from build123d import *

# Parameters (mm, degrees)
SKETCH_1_W          = 10
SKETCH_1_H          = 10
SKETCH_1_W_2        = 8
SKETCH_1_H_2        = 8
EXTRUDE_1_DEPTH     = 191.5
SKETCH_2_R          = 1.5
CUT_EXTRUDE_1_DEPTH = 11
SKETCH_3_R          = 1.5
CUT_EXTRUDE_2_DEPTH = 11


with BuildPart() as part:
    # 草图1 → 拉伸-薄壁1 (new body)
    with BuildSketch(Plane.XY):
        Rectangle(SKETCH_1_W, SKETCH_1_H)
        Rectangle(SKETCH_1_W_2, SKETCH_1_H_2, mode=Mode.SUBTRACT)
    extrude(amount=EXTRUDE_1_DEPTH)

    # 草图2 → 切除-拉伸1 (cut, through all)
    with BuildSketch(Plane.XZ.offset(5)):
        with Locations((0, 183.994446501)):
            Circle(SKETCH_2_R)
        with Locations((0, 29)):
            Circle(SKETCH_2_R)
        with Locations((0, 173.994446501)):
            Circle(SKETCH_2_R)
        with Locations((0, 100)):
            Circle(SKETCH_2_R)
        with Locations((0, 60)):
            Circle(SKETCH_2_R)
        with Locations((0, 146)):
            Circle(SKETCH_2_R)
        with Locations((0, 161)):
            Circle(SKETCH_2_R)
        Polygon((-5, 191.5), (5, 185.726497308), (5, 191.5), align=None)
    extrude(amount=-CUT_EXTRUDE_1_DEPTH, mode=Mode.SUBTRACT)

    # 草图3 → 切除-拉伸2 (cut, through all)
    with BuildSketch(Plane.ZY.offset(5)):
        with Locations((50, 0)):
            Circle(SKETCH_3_R)
        with Locations((120, 0)):
            Circle(SKETCH_3_R)
        with Locations((10, 0)):
            Circle(SKETCH_3_R)
        with Locations((155, 0)):
            Circle(SKETCH_3_R)
    extrude(amount=-CUT_EXTRUDE_2_DEPTH, mode=Mode.SUBTRACT)


solid = part.part
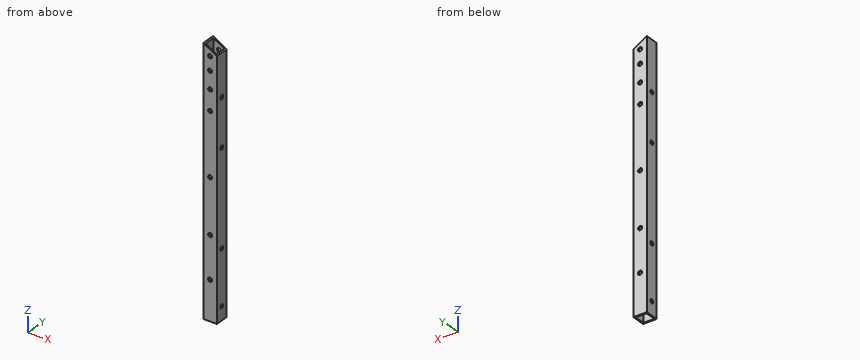
Source: CAD feature listing. Evaluate the final solid. Frame: model axes, mm. Round coordinates to 2 decimals unless told otherwise and drop trailing zeros. Loops run counter-clockwise (first coordinate to the right, second up) from the corner with the lowest first, then second, coordinate; pieces in that order, holes last. Notation, with made-up numbers: (88, 12) -> (119, 12) arc R20 cw to (119, 40) -> close; hole circle Ø8 at (88, 46). An arc over 180 degrees is marked (long way). Answer as a JSON object with one key per item and string values. Group by question number.
Q1. Ray query, line 1 (X direction, y = 3, z = 146); line 2 (X direction, y = 4.75, z = 161). Return the intervals inside material, ascending. Write a range as from..to.
Q2. Section query B-B (y = 0). State how many separate pieces and enclosed holes the cut face has, plus the area to 3 significant figures.
Q3. Section query A-A (z = 80.5). Output: boundary loops of the cut face in (x, y), plus the area to 3 significant figures.
Q4. Contact query for a flat-ended pin moving along its axis: P1, Ø2, axis at x = -2, y = 2.5, coming from the +Z side. Output: stop coordinate, or through.
Completed:
{
 "1": {"line 1": "-5..-4, 4..5", "line 2": "-5..-1.5, 1.5..5"},
 "2": {"separate pieces": "10", "enclosed holes": "0", "area": "353 mm²"},
 "3": {"outline": "(-5, -5) -> (5, -5) -> (5, 5) -> (-5, 5) -> close; hole (-4, -4) -> (4, -4) -> (4, 4) -> (-4, 4) -> close", "area": "36.0 mm²"},
 "4": {"P1": "through"}
}
